```python
from build123d import *

# Parameters (mm, degrees)
SKETCH005_W    = 0.4
SKETCH005_H    = 6.2
SKETCH003_W    = 0.4
SKETCH003_H    = 6.2
ARRAY001_COUNT = 4
ARRAY_COUNT    = 4
PAD_DEPTH      = 0.5
PAD001_DEPTH   = 13.17
FILLET_R       = 0.3
FILLET001_R    = 1
POCKET_DEPTH   = 0.2


with BuildPart() as revolution002:
    # Sketch005 → Revolution002 (revolve)
    with BuildSketch(Plane.XZ.offset(9.75)):
        with Locations((0.2, -3.1)):
            Rectangle(SKETCH005_W, SKETCH005_H)
    revolve(axis=Axis((0, -9.75, 0), (0, 0, 1)))


with BuildPart() as array001:
    # Sketch003 → Revolution001 (revolve)
    with BuildSketch(Plane.XZ.offset(-9.75)):
        with Locations((9.95, -3.1)):
            Rectangle(SKETCH003_W, SKETCH003_H)
    revolve(axis=Axis((9.75, 9.75, 0), (0, 0, -1)))

    # Array001: Array001 ×4 about axis
    array001_axis = Axis((0, 0, 0), (0, 0, 1))


with BuildPart() as array001_1:
    add(array001.part)
    for i in range(1, ARRAY001_COUNT):
        add(array001.part.rotate(array001_axis, i * 360 / ARRAY001_COUNT))


with BuildPart() as array:
    # Sketch002 → Revolution (revolve)
    with BuildSketch(Plane.XZ.offset(-5.75)):
        with BuildLine():
            Line((5.75, -0.65), (5.75, 0))
            Line((5.75, 0), (6.4, 0))
            ThreePointArc((5.75, -0.65), (6.2096194078, -0.4596194078), (6.4, 0))
        make_face()
    revolve(axis=Axis((5.75, 5.75, 0), (0, 0, -1)))

    # Array: Array ×4 about axis
    array_axis = Axis((0, 0, 0), (0, 0, 1))


with BuildPart() as array_1:
    add(array.part)
    for i in range(1, ARRAY_COUNT):
        add(array.part.rotate(array_axis, i * 360 / ARRAY_COUNT))


with BuildPart() as fusion002:
    # Sketch → Pad (new body)
    with BuildSketch(Plane.XY):
        with BuildLine():
            Line((-12, 13), (12, 13))
            ThreePointArc((13, 12), (12.7071067812, 12.7071067812), (12, 13))
            Line((13, 12), (13, -12))
            ThreePointArc((12, -13), (12.7071067812, -12.7071067812), (13, -12))
            Line((12, -13), (-13, -13))
            Line((-13, -13), (-13, 12))
            ThreePointArc((-12, 13), (-12.7071067812, 12.7071067812), (-13, 12))
        make_face()
    extrude(amount=PAD_DEPTH)

    # Sketch001 → Pad001 (new body)
    with BuildSketch(Plane.XY.offset(0.5)):
        with BuildLine():
            Line((-11.5, 12.5), (11.5, 12.5))
            ThreePointArc((12.5, 11.5), (12.2071067812, 12.2071067812), (11.5, 12.5))
            Line((12.5, 11.5), (12.5, -11.5))
            ThreePointArc((11.5, -12.5), (12.2071067812, -12.2071067812), (12.5, -11.5))
            Line((11.5, -12.5), (-11.5, -12.5))
            ThreePointArc((-12.5, -11.5), (-12.2071067812, -12.2071067812), (-11.5, -12.5))
            Line((-12.5, -11.5), (-12.5, 11.5))
            ThreePointArc((-11.5, 12.5), (-12.2071067812, 12.2071067812), (-12.5, 11.5))
        make_face()
    extrude(amount=PAD001_DEPTH)

    # Fillet
    fillet_edges = [fusion002.edges().sort_by_distance(p)[0] for p in [
        (12.5, 0, 0.5),
        (12.207107, -12.207107, 0.5),
        (0, -12.5, 0.5),
        (12.207107, 12.207107, 0.5),
        (-12.207107, -12.207107, 0.5),
        (0, 12.5, 0.5),
        (-12.207107, 12.207107, 0.5),
        (-12.5, 0, 0.5),
    ]]
    fillet(fillet_edges, radius=FILLET_R)

    # Fillet001
    fillet001_edges = [fusion002.edges().sort_by_distance(p)[0] for p in [
        (-12.5, 0, 13.67),
        (-12.207107, 12.207107, 13.67),
        (0, 12.5, 13.67),
        (12.207107, 12.207107, 13.67),
        (12.5, 0, 13.67),
        (12.207107, -12.207107, 13.67),
        (0, -12.5, 13.67),
        (-12.207107, -12.207107, 13.67),
    ]]
    fillet(fillet001_edges, radius=FILLET001_R)

    # Fusion: union Array
    add(array_1.part)

    # Fusion001: union Array001
    add(array001_1.part)

    # Sketch004 → Pocket (cut)
    with BuildSketch(Plane.XY.offset(13.67)):
        with BuildLine():
            Line((-4.5, 3), (4.5, 3))
            ThreePointArc((5, 2.5), (4.8535533906, 2.8535533906), (4.5, 3))
            Line((5, 2.5), (5, -2.5))
            ThreePointArc((4.5, -3), (4.8535533906, -2.8535533906), (5, -2.5))
            Line((4.5, -3), (-4.5, -3))
            ThreePointArc((-5, -2.5), (-4.8535533906, -2.8535533906), (-4.5, -3))
            Line((-5, -2.5), (-5, 2.5))
            ThreePointArc((-4.5, 3), (-4.8535533906, 2.8535533906), (-5, 2.5))
        make_face()
    extrude(amount=-POCKET_DEPTH, mode=Mode.SUBTRACT)

    # Fusion002: union Revolution002
    add(revolution002.part)


solid = fusion002.part
```
Input: part model. Units: mm. Frame: model coordinates. A direction names the side the tool comes from. Give positions to 0.01 mm unless a question says otherwise; leave off trailing zeros. Loops run counter-clockwise (first coordinate to the right, second up) from the corner with the lowest first, then second, coordinate; pieces in that order, holes last. Notation, with made-up numbers: (0.5, 79.25) -> (32.5, 79.25) arc R21 ccw to (32.5, 84.25) -> close; hole circle Ø6 at (-8, 13.5). An arc over 180 degrees is marked (long way). Use a Markdown table: item, result.
Q1. Section query A-A, the plane y = -9.75. Return the cut outline in (x, z), plus the area to 3 significant figures.
Entries:
| item | result |
|---|---|
| outline | (-13, 0) -> (-10.15, 0) -> (-10.15, -6.2) -> (-9.35, -6.2) -> (-9.35, 0) -> (-0.4, 0) -> (-0.4, -6.2) -> (0.4, -6.2) -> (0.4, 0) -> (9.35, 0) -> (9.35, -6.2) -> (10.15, -6.2) -> (10.15, 0) -> (13, 0) -> (13, 0.5) -> (12.8, 0.5) arc R0.3 cw to (12.5, 0.8) -> (12.5, 12.67) arc R1 ccw to (11.5, 13.67) -> (-11.5, 13.67) arc R1 ccw to (-12.5, 12.67) -> (-12.5, 0.8) arc R0.3 cw to (-12.8, 0.5) -> (-13, 0.5) -> close |
| area | 357 mm² |
Q2. Section query D-D, the plane x = 0. Return the cut outline in (y, z), plus the area to 3 significant figures.
Entries:
| item | result |
|---|---|
| outline | (-13, 0) -> (-10.15, 0) -> (-10.15, -6.2) -> (-9.35, -6.2) -> (-9.35, 0) -> (13, 0) -> (13, 0.5) -> (12.8, 0.5) arc R0.3 cw to (12.5, 0.8) -> (12.5, 12.67) arc R1 ccw to (11.5, 13.67) -> (3, 13.67) -> (3, 13.47) -> (-3, 13.47) -> (-3, 13.67) -> (-11.5, 13.67) arc R1 ccw to (-12.5, 12.67) -> (-12.5, 0.8) arc R0.3 cw to (-12.8, 0.5) -> (-13, 0.5) -> close |
| area | 346 mm² |
Q3. Section query B-B, the plane z = -2. Return the cut outline in (x, y).
Entries:
| item | result |
|---|---|
| outline | circle Ø0.8 at (-9.75, -9.75); circle Ø0.8 at (-9.75, 9.75); circle Ø0.8 at (0, -9.75); circle Ø0.8 at (9.75, -9.75); circle Ø0.8 at (9.75, 9.75) |
Q4. Ray query, probe 1 along Y at (x, z) = (9.75, -4); probe 2 along Z at (x, y) = (10.5, 0.5); probe 3 along Z at (x, y) = (-0.25, -1.5). Return the intervals inside material, ascending. Write a range as from..to.
Entries:
| item | result |
|---|---|
| probe 1 | y = -10.15..-9.35, 9.35..10.15 |
| probe 2 | z = 0..13.67 |
| probe 3 | z = 0..13.47 |
Q5. Section query C-C, the plane z = 6.75. Return the cut outline in (x, y).
Entries:
| item | result |
|---|---|
| outline | (-12.5, -11.5) arc R1 ccw to (-11.5, -12.5) -> (11.5, -12.5) arc R1 ccw to (12.5, -11.5) -> (12.5, 11.5) arc R1 ccw to (11.5, 12.5) -> (-11.5, 12.5) arc R1 ccw to (-12.5, 11.5) -> close |
Q6. Access query for faces 1 (the cylindrical face through (-12.199, 12.215, 6.652)), 2 (the cylindrical face through (12.199, -12.215, 6.652)), 3 (the flat face through (0, 0, 13.47)), 4 (the cylindrical face through (-12.215, -12.199, 6.652)), 5 (the flat face through (12.5, 0, 7)). Directions: +Z, -Z, +X, -X, +Y, -Y. A direction counts if a zero-diameter tool reaches every point of the face in a straight line with its end or side. Return the directions, or none.
Entries:
| item | result |
|---|---|
| face 1 | +Z, -X, +Y |
| face 2 | +Z, +X, -Y |
| face 3 | +Z |
| face 4 | +Z, -X, -Y |
| face 5 | +Z, +X, +Y, -Y |
Q7. First-contact query: P1, Ø8, axis at y = -2.5, z = 11, coming from the -X side; P2, Ø4, axis at x = 7, y = 10.5, coming from the -Z side; P3, Ø6, axis at y = -2, z = 8.5, coming from the +X side. Flat tips, straight axial feed; report the tip coordinate or a pass-through.
Entries:
| item | result |
|---|---|
| P1 | stops at x = -12.5 |
| P2 | stops at z = 0 |
| P3 | stops at x = 12.5 |
Q8. Pull-direction query (X, two-part tool) for faces 6 (the cylindrical face through (-12.215, 0.161, 13.369)), 7 (the cylindrical face through (0.185, -10.105, -3.057)), 8 (the cylindrical face through (12.215, 12.199, 6.652)); classes: pulls with the +X half, pulls with the -X half, needs draft (parallel to the pull), parting line crosses it, or undercut.
Entries:
| item | result |
|---|---|
| face 6 | pulls with the -X half |
| face 7 | undercut |
| face 8 | pulls with the +X half |
